Drawing for the job (mm, zero at the part's lowest x, y, z). A direction names the side the tool comes from. Give positions to 0.01 mm unless a question says otherwise; leave off trailing zeros. Order: outer loops, then holes, each group sorted by start corner. A loop starts at its lowest first (then second) coordinate and runs counter-clockwise, first axis right, second up. Notation, with made-up numbers: (57.5, 65) - (69.5, 65) arc R35 ccw to (69.5, 104) - close; hole circle Ø10 at (24, 81.25). An arc over 180 degrees is marked (long way). One line per item, written item: value.
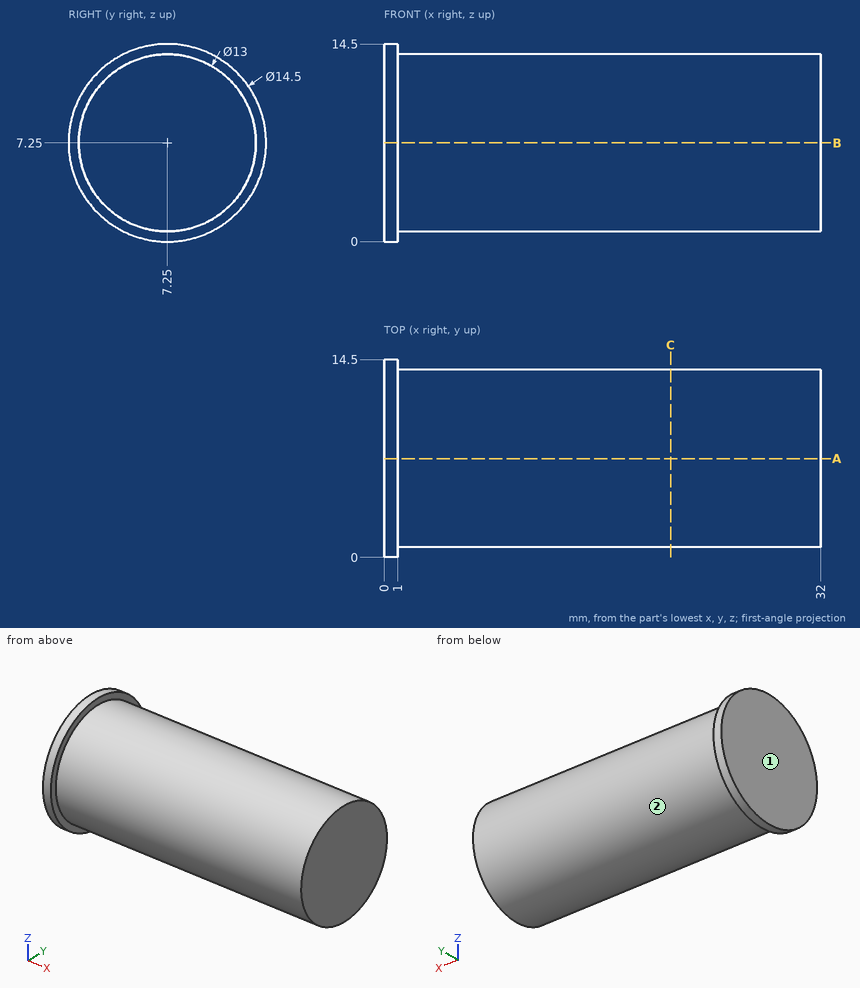
1) Which spindle directions (+Z, -Z, +X, -X, +Y, -Y) get a long thin tool onto all of the face, cutting with end or side? Do the marked faces 1 and 2. Say none if no direction does.
Outcome:
face 1: +Z, -Z, -X, +Y, -Y
face 2: +X
2) Cut at C-C, the plane x = 21. Give the cut face in (y, z).
Outcome:
outline: circle Ø13 at (7.25, 7.25)
3) Cut at A-A, the plane y = 7.25. Give the cut face in (x, z), then the cut area to 4 significant figures.
Outcome:
outline: (0, 0) - (1, 0) - (1, 0.75) - (32, 0.75) - (32, 13.75) - (1, 13.75) - (1, 14.5) - (0, 14.5) - close
area: 417.5 mm^2
4) Drill centre lines: line 1 along Y through (x, z) = (16, 7.5); line 2 along Y through (x, z) = (20.5, 4); line 3 along Z through (x, y) = (28.5, 5). Where is each one in solid material? Low to high. Write a range as from..to.
Outcome:
line 1: y = 0.75..13.75
line 2: y = 1.62..12.88
line 3: z = 1.15..13.35
5) Pin check, flat tips, straight feed: pin 1 (4 mm diameter, centred on x = 8, y = 6.5, fed in from -Z); pin 2 (4 mm diameter, centred on x = 5.5, y = 4, fed in from -Z); pin 3 (1.5 mm diameter, centred on x = 18, z = 2.5, fed in from -Y). Stop position of each tip, or through.
Outcome:
pin 1: stops at z = 0.75
pin 2: stops at z = 0.87
pin 3: stops at y = 2.13
